The listing builds one solid part. Answer for the finished solid, in the listing's coordinates (mm). A direction names the side the tool comes from. Round coordinates to 2 decimals unless told otherwise and drop trailing zeros. Write each loop counter-clockwise with the first axis right and the second up, starting at its lowest first coordinate (ties: lowest second). Pieces come first, ordered by that corner, then holes. Notation, with made-up numbers: (-19.5, 61.5) - (-6.5, 61.5) arc R37 cw to (-6.5, 98.5) - close; hole circle Ø3 at (10.5, 46). An arc over 180 degrees is marked (long way). Return JSON: item names as keys, results as strings. Group by question number.
from build123d import *

# Parameters (mm, degrees)
ARRAY005_X_COUNT = 5
ARRAY005_X_PITCH = 2.77
ARRAY004_X_COUNT = 4
ARRAY004_X_PITCH = 2.77
SKETCH016_R      = 0.7
PAD006_DEPTH     = 0.5
ARRAY_X_COUNT    = 5
ARRAY_X_PITCH    = 2.77
SKETCH017_R      = 0.7
PAD007_DEPTH     = 0.5
ARRAY001_X_COUNT = 4
ARRAY001_X_PITCH = 2.77
PAD004_DEPTH     = 3.45
PAD005_DEPTH     = 2
FILLET007_R      = 0.7


with BuildPart() as array005:
    # Sketch020 → Revolution004 (revolve)
    with BuildSketch(Plane.XZ):
        with BuildLine():
            Line((0, 5), (0, -10.75))
            ThreePointArc((0, -10.75), (0.212132, -10.662132), (0.3, -10.45))
            Line((0.3, -10.45), (0.3, -2))
            Line((0.3, -2), (0.5, -2))
            Line((0.5, -2), (0.5, 4.5))
            ThreePointArc((0.5, 4.5), (0.353553, 4.853553), (0, 5))
        make_face()
    revolve(axis=Axis((0, 0, 0), (0, 0, 1)))


with BuildPart() as array005_1:
    # Body011 placement: moved
    add(array005.part.moved(Location((-5.54, 1.42, 0))))

    # Array005 X: Array005 ×5


with BuildPart() as array005_2:
    add(array005_1.part)
    with Locations(*[(i * ARRAY005_X_PITCH, 0, 0) for i in range(1, ARRAY005_X_COUNT)]):
        add(array005_1.part)


with BuildPart() as fusion001:
    # Sketch021 → Revolution005 (revolve)
    with BuildSketch(Plane.XZ):
        with BuildLine():
            Line((0, 5), (0, -10.75))
            ThreePointArc((0, -10.75), (0.212132, -10.662132), (0.3, -10.45))
            Line((0.3, -10.45), (0.3, -2))
            Line((0.3, -2), (0.5, -2))
            Line((0.5, -2), (0.5, 4.5))
            ThreePointArc((0.5, 4.5), (0.353553, 4.853553), (0, 5))
        make_face()
    revolve(axis=Axis((0, 0, 0), (0, 0, 1)))


with BuildPart() as fusion001_1:
    # Body012 placement: moved
    add(fusion001.part.moved(Location((-4.155, -1.42, 0))))

    # Array004 X: Fusion001 ×4


with BuildPart() as fusion001_2:
    add(fusion001_1.part)
    with Locations(*[(i * ARRAY004_X_PITCH, 0, 0) for i in range(1, ARRAY004_X_COUNT)]):
        add(fusion001_1.part)

    # Fusion001: union Array005
    add(array005_2.part)


with BuildPart() as array:
    # Sketch016 → Pad006 (new body)
    with BuildSketch(Plane.XY):
        Circle(SKETCH016_R)
    extrude(amount=-PAD006_DEPTH)


with BuildPart() as array_1:
    # Body007 placement: moved
    add(array.part.moved(Location((-5.54, 1.42, -5.45))))

    # Array X: Array ×5


with BuildPart() as array_2:
    add(array_1.part)
    with Locations(*[(i * ARRAY_X_PITCH, 0, 0) for i in range(1, ARRAY_X_COUNT)]):
        add(array_1.part)


with BuildPart() as array001:
    # Sketch017 → Pad007 (new body)
    with BuildSketch(Plane.XY):
        Circle(SKETCH017_R)
    extrude(amount=-PAD007_DEPTH)


with BuildPart() as array001_1:
    # Body008 placement: moved
    add(array001.part.moved(Location((-4.155, -1.42, -5.45))))

    # Array001 X: Array001 ×4


with BuildPart() as array001_2:
    add(array001_1.part)
    with Locations(*[(i * ARRAY001_X_PITCH, 0, 0) for i in range(1, ARRAY001_X_COUNT)]):
        add(array001_1.part)


with BuildPart() as cut:
    # Sketch014 → Pad004 (new body)
    with BuildSketch(Plane.XY):
        with BuildLine():
            Line((-5.72, 5), (5.72, 5))
            ThreePointArc((9.068211, 1.008831), (8.324801, 3.78518), (5.72, 5))
            Line((9.068211, 1.008831), (8.503211, -2.191169))
            ThreePointArc((5.155, -5), (7.34018, -4.204801), (8.503211, -2.191169))
            Line((5.155, -5), (-5.155, -5))
            ThreePointArc((-8.503211, -2.191169), (-7.34018, -4.204801), (-5.155, -5))
            Line((-8.503211, -2.191169), (-9.068211, 1.008831))
            ThreePointArc((-5.72, 5), (-8.324801, 3.78518), (-9.068211, 1.008831))
        make_face()
    extrude(amount=-PAD004_DEPTH)

    # Sketch015 (on Face10 of Pad004) → Pad005 (join)
    with BuildSketch(Plane(origin=(0, 0, -3.45), x_dir=(1, 0, 0), z_dir=(0, 0, -1))):
        with BuildLine():
            Line((-5.155, 4.2), (5.155, 4.2))
            ThreePointArc((7.715397, 2.05207), (6.82602, 3.591906), (5.155, 4.2))
            Line((7.715397, 2.05207), (8.280397, -1.14793))
            ThreePointArc((5.72, -4.2), (7.711906, -3.27102), (8.280397, -1.14793))
            Line((5.72, -4.2), (-5.72, -4.2))
            ThreePointArc((-8.280397, -1.14793), (-7.711906, -3.27102), (-5.72, -4.2))
            Line((-8.280397, -1.14793), (-7.715397, 2.05207))
            ThreePointArc((-5.155, 4.2), (-6.82602, 3.591906), (-7.715397, 2.05207))
        make_face()
    extrude(amount=PAD005_DEPTH)

    # Fillet007
    fillet007_edges = [cut.edges().sort_by_distance(p)[0] for p in [
        (-8.785711, -0.591169, -3.45),
    ]]
    fillet(fillet007_edges, radius=FILLET007_R)

    # Fusion: union Array, Array001
    add(array_2.part)
    add(array001_2.part)

    # Cut: cut Fusion001
    add(fusion001_2.part, mode=Mode.SUBTRACT)


solid = cut.part
(1) For faces 1 (the cylindrical face through (-2.084, -1.389, -5.696)), 2 (the cylindrical face through (6.845, -3.575, -4.436)), 3 (the cylindrical face through (-3.693, -1.612, -0.986)), determine the directions among +Z, -Z, +X, -X, +Y, -Y from which every point of the face is accessible in a straight line to the end or side of a thin tool.
(2) Consider line 1 (Z direction, x = 7.25, y = 2.5); line 2 (X direction, y = 1.75, z = -1.3); line 3 (X direction, y = -2, z = -5.6). Determine where each line is inside the solid, lowest interval first.
(3) Find section D-D (x = 4.25). Write down the section's boundary in (y, z).
(4) Find section A-A (x = -2.77). Write down the section's boundary in (y, z).
(5) Find section B-B (z = -4.8). State how many separate pieces and enclosed holes the cut face has, plus the area to 3 significant figures.
(6) Flat-ended cylindrical pins translate along their axes: pin 1 (0.5 mm diameter, centred on x = 1.5, y = -1.5, fed in from +Z); pin 2 (1.6 mm diameter, centred on x = -1, z = -5, fed in from -Y); pin 3 (2 mm diameter, centred on x = 2.5, z = -5, fed in from +Y). Find the tip coordinate at first contact, or state that the pin passes through.
(7) Determine the mould class of faces 4 (the flat face through (-8, -0.43, -4.44)), 5 (the cylindrical face through (-2.308, 1.228, -0.986)), 6 (the flat face through (3, 1, -5.95)) for opening direction Y: +Y half, -Y half, draft (parallel to the pull), parting line (faces both ways), or undercut.
Check sheet entries:
{
 "1": {"face 1": "-Z", "face 2": "-Z, +X, -Y", "face 3": "+Z"},
 "2": {"line 1": "z = -5.45 to 0", "line 2": "x = -9.12 to -5.92, -5.16 to -3.15, -2.39 to -0.38, 0.38 to 2.39, 3.15 to 5.16, 5.92 to 9.12", "line 3": "x = -4.55 to -3.76, -1.78 to -0.99, 0.99 to 1.78, 3.76 to 4.55"},
 "3": {"outline": "(-5, -2.75) arc R0.7 ccw to (-4.3, -3.45) - (-4.2, -3.45) - (-4.2, -5.45) - (-2.11, -5.45) - (-2.11, -5.95) - (-1.7, -5.95) - (-1.7, -2) - (-1.91, -2) - (-1.91, 0) - (-5, 0) - close; (-1.14, -5.95) - (-0.73, -5.95) - (-0.73, -5.45) - (4.2, -5.45) - (4.2, -3.45) - (4.3, -3.45) arc R0.7 ccw to (5, -2.75) - (5, 0) - (-0.93, 0) - (-0.93, -2) - (-1.14, -2) - close"},
 "4": {"outline": "(-5, -2.75) arc R0.7 ccw to (-4.3, -3.45) - (-4.2, -3.45) - (-4.2, -5.45) - (0.72, -5.45) - (0.72, -5.95) - (1.12, -5.95) - (1.12, -2) - (0.92, -2) - (0.92, 0) - (-5, 0) - close; (1.72, -5.95) - (2.12, -5.95) - (2.12, -5.45) - (4.2, -5.45) - (4.2, -3.45) - (4.3, -3.45) arc R0.7 ccw to (5, -2.75) - (5, 0) - (1.92, 0) - (1.92, -2) - (1.72, -2) - close"},
 "5": {"separate pieces": "1", "enclosed holes": "9", "area": "127 mm^2"},
 "6": {"pin 1": "stops at z = -2", "pin 2": "stops at y = -4.2", "pin 3": "stops at y = 4.2"},
 "7": {"face 4": "-Y half", "face 5": "undercut", "face 6": "draft"}
}
